Build history of the part. All positions in model axes, mm. Round coordinates to 2 decimals unless told otherwise and drop trailing zeros. Loops run counter-clockwise (first coordinate to the right, second up) from the corner with the lowest first, then second, coordinate; pieces in that order, holes last. Notation, with made-up numbers: (7, -23) - (37, -23) arc R27 ccw to (37, 1) - close; hole circle Ø9 at (64, 65.25). An arc over 180 degrees is marked (long way). Use a Markdown table: item, result.
from build123d import *

# Parameters (mm, degrees)
SKETCH049_R     = 151.5
PAD_DEPTH       = 8
SKETCH050_R     = 145.3
PAD008_DEPTH    = 3.8
SKETCH051_R     = 1
SKETCH051_R_2   = 3
POCKET_DEPTH    = 8
SKETCH052_R     = 38
POCKET005_DEPTH = 11.801


with BuildPart() as part:
    # Sketch049 → Pad (new body)
    with BuildSketch(Plane.XY):
        Circle(SKETCH049_R)
    extrude(amount=PAD_DEPTH)

    # Sketch050 (on Face3 of Pad) → Pad008 (join)
    with BuildSketch(Plane.XY.offset(8)):
        Circle(SKETCH050_R)
    extrude(amount=PAD008_DEPTH)

    # Sketch051 (on Face5 of Pad008) → Pocket (cut)
    with BuildSketch(Plane.XY.offset(11.8)):
        with Locations((-38, -113.75)):
            Circle(SKETCH051_R)
        with Locations((-71.827358, -98.861877)):
            Circle(SKETCH051_R)
        with Locations((38, -113.75)):
            Circle(SKETCH051_R)
        with Locations((71.827358, -98.861877)):
            Circle(SKETCH051_R)
        with Locations((38, 14.25)):
            Circle(SKETCH051_R)
        with Locations((-38, 14.25)):
            Circle(SKETCH051_R)
        with Locations((-116.219106, 37.761877)):
            Circle(SKETCH051_R)
        with Locations((116.219106, 37.761877)):
            Circle(SKETCH051_R)
        with Locations((0, 139.3)):
            Circle(SKETCH051_R_2)
    extrude(amount=-POCKET_DEPTH, mode=Mode.SUBTRACT)

    # Sketch052 (on Face5 of Pad008) → Pocket005 (cut, through all)
    with BuildSketch(Plane.XY.offset(11.8)):
        with Locations((0, -75.75)):
            Circle(SKETCH052_R)
    extrude(amount=-POCKET005_DEPTH, mode=Mode.SUBTRACT)


with BuildPart() as part_1:
    # Body placement: moved
    add(part.part.moved(Location((0, 150, 0))))


solid = part_1.part
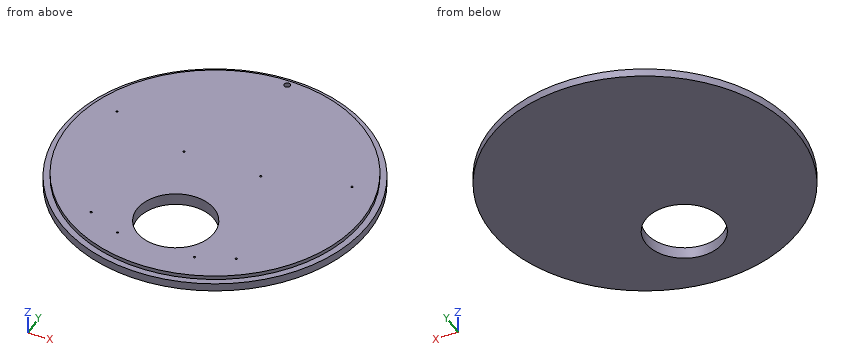
Q1. Cut at B-B, the plane y = 19. List the corners of the cut face in (x, z).
Results found:
| item | result |
|---|---|
| outline | (-76.1, 0) - (76.1, 0) - (76.1, 8) - (62.86, 8) - (62.86, 11.8) - (-62.86, 11.8) - (-62.86, 8) - (-76.1, 8) - close |
Q2. Cut at A-A, the plane x = 32. List the corners of the cut face in (y, z), plus the area to 3 significant figures.
Results found:
| item | result |
|---|---|
| outline | (1.92, 0) - (53.76, 0) - (53.76, 11.8) - (8.27, 11.8) - (8.27, 8) - (1.92, 8) - close; (94.74, 0) - (298.08, 0) - (298.08, 8) - (291.73, 8) - (291.73, 11.8) - (94.74, 11.8) - close |
| area | 2,960 mm2 |
Q3. Probe line 1 (Z direction, x = -129, y = 220.5); line 2 (Y direction, x = -8.5, z = 9); line 3 (X direction, y = 59, z = 0.75). List the from-to ranges inside material, lowest first.
Results found:
| item | result |
|---|---|
| line 1 | z = 0 to 8 |
| line 2 | y = 4.95 to 37.21, 111.29 to 295.05 |
| line 3 | x = -121.12 to -34.81, 34.81 to 121.12 |
Q4. Cut at C-C, the plane x = 67. List the corners of the cut face in (y, z).
Results found:
| item | result |
|---|---|
| outline | (14.12, 0) - (285.88, 0) - (285.88, 8) - (278.93, 8) - (278.93, 11.8) - (21.07, 11.8) - (21.07, 8) - (14.12, 8) - close |
Q5. Drop flat-ended pins along their axis: pin 1 (1.8 mm diameter, centred on x = 116.22, y = 187.76, fed in from +Z); pin 2 (2.5 mm diameter, centred on x = -71.83, y = 51.14, fed in from -Z); pin 3 (5 mm diameter, centred on x = 73.5, z = 10, fed in from -Y); pin 4 (6 mm diameter, centred on y = 37.5, z = 3.5, fed in from +X). Give the stop position or say it passes through.
Results found:
| item | result |
|---|---|
| pin 1 | stops at z = 3.8 |
| pin 2 | stops at z = 0 |
| pin 3 | stops at y = 16.7 |
| pin 4 | stops at x = 104.7 |
